Read the model definition and answer for the solid it produces. Units are mm, in the model's axes. Face numbers are marked on the shaded views. Give positions to 0.01 mm unless a question says otherwise; leave off trailing zeros. Order: outer loops, then holes, each group sorted by start corner. A loop starts at its lowest first (then second) coordinate and runs counter-clockwise, first axis right, second up. Notation, with made-up numbers: (88, 31.5) - (140, 31.5) arc R23 ccw to (140, 67.5) - close; hole circle Ø10 at (54, -2). An arc over 180 degrees is marked (long way). Use a Markdown table: item, result. Add a question column.
1. For a pull along X with two mould halves and no side action, classify the marked faces 1, 2 and 3 as released by +X, released by -X, zero draft, split by the parting line, or undercut.
2. A cutting plane is placed at C-C on x = -44.5. Determine the outline of the cut face in (y, z), and give its area (3 significant figures).
3. A cutting plane is placed at A-A on x = 0. Determine the outline of the cut face in (y, z).
4. A cutting plane is placed at B-B on z = 0. Determine the outline of the cut face in (x, y), and give its area (3 significant figures).
5. A cutting plane is placed at D-D on y = 43.5. Determine the outline of the cut face in (x, z).
6. Consider L1, parallel to X at y = 37, z = 0; L2, parallel to Y at x = 14, z = -7; L3, parallel to X at y = 9, z = -30. Determine where each line is inside the solid, lowest interval first.
7. Flat-ended cylindrical pins translate along their axes: P1, Ø10, axis at x = 36, y = 37, coming from the +Z side; P2, Ø12, axis at y = 39.5, z = -21.5, coming from the +X side; P3, Ø10, axis at y = 22, z = 30.5, coming from the +X side; P4, Ø2, axis at x = 44, z = -3, coming from the -Y side. Find the tip coordinate at first contact, or state that the pin passes through.
```python
from build123d import *

# Parameters (mm, degrees)
SKETCH1_R           = 62.5
SKETCH1_R_2         = 59.5
BOSS_EXTRUDE1_DEPTH = 3
SKETCH1_3_R         = 62.5
SKETCH1_3_R_2       = 59.5
BOSS_EXTRUDE2_DEPTH = 50
CUT_EXTRUDE1_DEPTH  = 50


with BuildPart() as part:
    # Sketch1 → Boss-Extrude1 (new body)
    with BuildSketch(Plane(origin=(0, 0, 0), x_dir=(1, 0, 0), z_dir=(0, 1, 0))):
        with Locations(Location((0, 0, 0), (0, 0, 270))):
            Circle(SKETCH1_R)
        Circle(SKETCH1_R_2, mode=Mode.SUBTRACT)
        Circle(SKETCH1_R_2)
    extrude(amount=BOSS_EXTRUDE1_DEPTH)

    # Sketch1_3 → Boss-Extrude2 (add)
    with BuildSketch(Plane(origin=(0, 0, 0), x_dir=(1, 0, 0), z_dir=(0, 1, 0))):
        with Locations(Location((0, 0, 0), (0, 0, 270))):
            Circle(SKETCH1_3_R)
        with Locations(Location((0, 0, 0), (0, 0, 270))):
            Circle(SKETCH1_3_R_2, mode=Mode.SUBTRACT)
    extrude(amount=BOSS_EXTRUDE2_DEPTH)

    # Sketch2 → Cut-Extrude1 (cut)
    with BuildSketch(Plane.XZ):
        with BuildLine():
            Line((-2.122524784, -48.573163327), (-2.122524784, -34.368574388))
            ThreePointArc((-2.122524784, -34.368574388), (0, -32.246049604), (2.122524784, -34.368574388))
            Line((2.122524784, -34.368574388), (2.122524784, -48.573163327))
            ThreePointArc((2.122524784, -48.573163327), (0, -50.695688111), (-2.122524784, -48.573163327))
        make_face()
    extrude(amount=-CUT_EXTRUDE1_DEPTH, mode=Mode.SUBTRACT)


solid = part.part
```
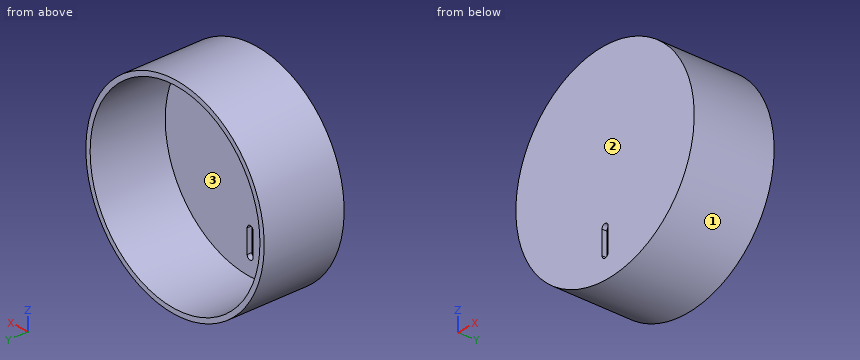
Output values:
| question | item | result |
|---|---|---|
| 1 | face 1 | split by the parting line |
| 1 | face 2 | zero draft |
| 1 | face 3 | undercut |
| 2 | outline | (0, -43.89) - (50, -43.89) - (50, -39.5) - (3, -39.5) - (3, 39.5) - (50, 39.5) - (50, 43.89) - (0, 43.89) - close |
| 2 | area | 676 mm² |
| 3 | outline | (0, -62.5) - (50, -62.5) - (50, -59.5) - (3, -59.5) - (3, -50.7) - (0, -50.7) - close; (0, -32.25) - (3, -32.25) - (3, 59.5) - (50, 59.5) - (50, 62.5) - (0, 62.5) - close |
| 4 | outline | (-62.5, 0) - (62.5, 0) - (62.5, 50) - (59.5, 50) - (59.5, 3) - (-59.5, 3) - (-59.5, 50) - (-62.5, 50) - close |
| 4 | area | 657 mm² |
| 5 | outline | circle Ø125 at (0, 0); hole circle Ø119 at (0, 0) |
| 6 | L1 | -62.5 to -59.5, 59.5 to 62.5 |
| 6 | L2 | 0 to 3 |
| 6 | L3 | -54.83 to -51.38, 51.38 to 54.83 |
| 7 | P1 | z = 54.27 |
| 7 | P2 | x = 60.55 |
| 7 | P3 | x = 57.06 |
| 7 | P4 | y = 0 |
